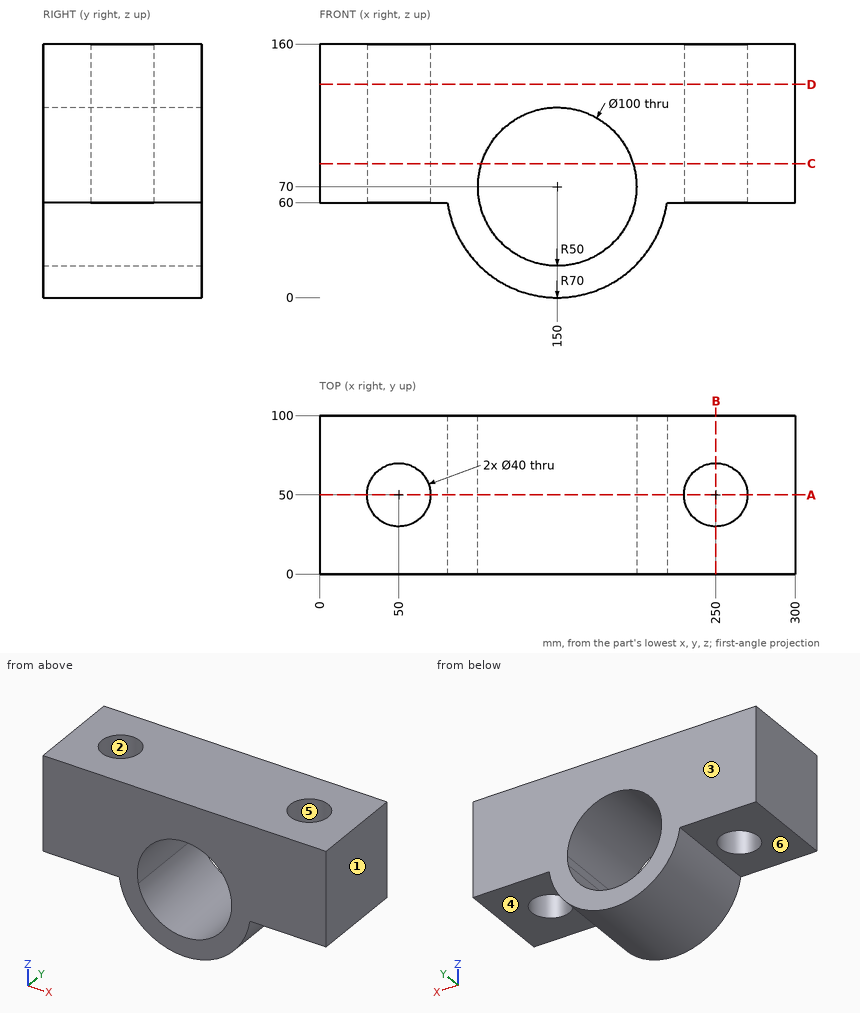
Could you check a few things on this drawing? It's one solid part, dimensions in mm from its lowest x, y, z. A direction names the side the tool comes from. Coordinates: 2 decimals unless noted, no trailing zeros. Order: outer loops, then holes, each group sorted by start corner. A loop starts at its lowest first (then second) coordinate and runs counter-clockwise, first axis right, second up. Notation, with made-up numbers: (37.25, 31) - (74.25, 31) arc R24 ccw to (74.25, 49) - close; hole circle Ø1 at (18.25, 59.25). An arc over 180 degrees is marked (long way). One line per question, with ' | ' between items.
(1) If I drill on L1, parallel to Y at x = 250, z = 95; L2, parallel to X at y = 38, z = 92; L3, parallel to X at y = 65, z = 70, over which ranges is the centre line in solid material (lowest first)?
Report:
L1: y = 0 to 30, 70 to 100 | L2: x = 0 to 34, 66 to 105.1, 194.9 to 234, 266 to 300 | L3: x = 0 to 36.77, 63.23 to 100, 200 to 236.77, 263.23 to 300
(2) If we mould it in two halves opening along Y, with no side actions, what happens to the marked faces 1, 2 and 3? For each: pulls with the +Y half, pulls with the -Y half, needs draft (parallel to the pull), parting line crosses it, or undercut.
Report:
face 1: needs draft | face 2: undercut | face 3: pulls with the +Y half
(3) Suppose I cut it at D-D on z = 134.5. List the corners of the cut face in (x, y) for me, and give its area (3 significant figures).
Report:
outline: (0, 0) - (300, 0) - (300, 100) - (0, 100) - close; hole circle Ø40 at (50, 50); hole circle Ø40 at (250, 50) | area: 27,500 mm2
(4) For the marked faces 4, 5 and 6, which set-ups out of +Z, -Z, +X, -X, +Y, -Y let a thin tool reach every point of the face, with its end or its side?
Report:
face 4: -Z, +X, +Y, -Y | face 5: +Z, -Z | face 6: -Z, -X, +Y, -Y
(5) Suppose I cut it at C-C on z = 84.5. List the corners of the cut face in (x, y) for me, and give its area (3 significant figures).
Report:
outline: (0, 0) - (102.15, 0) - (102.15, 100) - (0, 100) - close; (197.85, 0) - (300, 0) - (300, 100) - (197.85, 100) - close; hole circle Ø40 at (50, 50); hole circle Ø40 at (250, 50) | area: 17,900 mm2
(6) Suppose I cut it at B-B on x = 250. List the corners of the cut face in (y, z) for me, and give its area (3 significant figures).
Report:
outline: (0, 60) - (30, 60) - (30, 160) - (0, 160) - close; (70, 60) - (100, 60) - (100, 160) - (70, 160) - close | area: 6,000 mm2
(7) Will these pins go through, and if not, where does the flat tip stop? pin 1 (12 mm diameter, centred on x = 136, y = 47.5, fed in from -Z); pin 2 (24 mm diameter, centred on x = 43.5, y = 72.5, fed in from -Z); pin 3 (24 mm diameter, centred on x = 250, y = 50, fed in from -Z); pin 4 (2 mm diameter, centred on y = 27, z = 29, fed in from -X).
Report:
pin 1: stops at z = 0.46 | pin 2: stops at z = 60 | pin 3: passes through | pin 4: stops at x = 92.55
(8) Suppose I cut it at A-A on y = 50. List the corners of the cut face in (x, z) for me, and give its area (3 significant figures).
Report:
outline: (0, 60) - (30, 60) - (30, 160) - (0, 160) - close; (70, 60) - (80.72, 60) arc R70 ccw to (219.28, 60) - (230, 60) - (230, 160) - (70, 160) - close; (270, 60) - (300, 60) - (300, 160) - (270, 160) - close; hole (198.99, 60) arc R50 ccw to (200, 70) arc R50 ccw (long way) to start | area: 20,400 mm2
